Check sheet for the modelled part. Datum: model origin and axes. Units: mm. Coordinates: 2 decimals unless noted, no trailing zeros. Write each loop counter-clockwise with the first axis right and the second up, starting at its lowest first coordinate (ties: lowest second). Pieces come first, ordered by that corner, then holes. Notation, with made-up numbers: M -31,10.25 L 2,10.25 A22 ccw 2,49.25 Z; hole C 45,64 d10. An arc over 180 degrees is marked long. Answer as CSV lines item,"result". Start each with the question number.
Q1. Sectioned sample at C-C, the plane x = -4.75. Record the cut outline in (y, z).
Q2. Thickness scan on line 1 along Z through (x, y) = (-4, 3.5); line 2 along X through (y, z) = (0, -30.5) (3 decimals). Record the ranges inside material, lowest first. Write a range as from..to.
Q3. Sectioned sample at B-B, the plane z = -45. Record the cut outline in (x, y) (3 decimals).
Q4. Sectioned sample at A-A, the plane y = 0. Record the cut outline in (x, z) (1 decimal).
Q5. Depth check by flat-ended pin: pin 1 Ø1.8 at (y, z) = (0.5, -1.5) entering from -X; pin 2 Ø4 at (y, z) = (3.5, -17) entering from -X; pin 3 Ø1.1 at (y, z) = (-0.5, -1.5) entering from +X. Enter the tip coordinate at first touch or a pass-through.
from build123d import *

# Parameters (mm, degrees)
SKETCH1_W          = 47.625
SKETCH1_H          = 3.175
CHAMFER1_SIZE      = 0.9525
CUT_EXTRUDE2_DEPTH = 2.34696


with BuildPart() as part:
    # Sketch1 → Revolve1 (revolve)
    with BuildSketch(Plane(origin=(0, 0, 0), x_dir=(0, 0, -1), z_dir=(1, 0, 0))):
        with Locations((27.1653, 1.5875)):
            Rectangle(SKETCH1_W, SKETCH1_H)
    revolve(axis=Axis((0, 0, -50.9778), (0, 0, 1)))

    # Chamfer1
    chamfer1_edges = [part.edges().sort_by_distance(p)[0] for p in [
        (0, -3.175, -50.9778),
    ]]
    chamfer(chamfer1_edges, length=CHAMFER1_SIZE)

    # Sketch7 → Revolve2 (revolve)
    with BuildSketch(Plane(origin=(0, 0, 0), x_dir=(0, 0, -1), z_dir=(1, 0, 0)), mode=Mode.PRIVATE) as revolve2_sk:
        with BuildLine():
            Line((2.84988, 5.5499), (3.3528, 5.5499))
            Line((3.3528, 5.5499), (3.3528, 0))
            Line((3.3528, 0), (0, 0))
            Line((0, 0), (0, 3.175))
            ThreePointArc((0, 3.175), (1.235921075, 4.58927271), (2.84988, 5.5499))
        make_face()
    revolve(revolve2_sk.sketch.rotate(Axis((0, 0, 0), (0, 0, -1)), 180), axis=Axis((0, 0, 0), (0, 0, -1)))

    # Sketch5 → Cut-Extrude2 (cut)
    with BuildSketch(Plane.XY):
        Polygon((1.984375, -1.14567944), (1.984375, 1.14567944), (0, 2.291358881), (-1.984375, 1.14567944), (-1.984375, -1.14567944), (0, -2.291358881), align=None)
    extrude(amount=-CUT_EXTRUDE2_DEPTH, mode=Mode.SUBTRACT)

    # Cut-Extrude3 cone 1 section (on through the dimple's axis) → Cut-Extrude3 (revolve, cut)
    with BuildSketch(Plane(origin=(0, 0, 0), x_dir=(0, -1, 0), z_dir=(1, 0, 0))):
        Polygon((0, 0), (2.291358881, 0), (0, 2.291358881), align=None)
    revolve(axis=Axis((0, 0, 0), (0, 0, -1)), mode=Mode.SUBTRACT)


solid = part.part
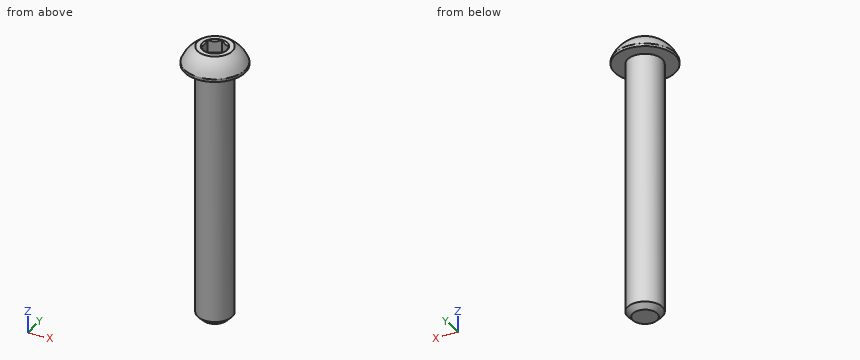
Output:
1,outline,"M -2.87,-3.35 L 2.87,-3.35 L 2.87,-2.85 A3.62 ccw -2.87,-2.85 Z"
2,line 1,"z = -3.35..-2.33"
2,line 2,"x = -3.175..3.175"
3,outline,"C 0,0 d6.35"
4,outline,"M -5.5,-3.4 L -3.2,-3.4 L -3.2,-50 L -2.2,-51 L 2.2,-51 L 3.2,-50 L 3.2,-3.4 L 5.5,-3.4 L 5.5,-2.8 A6 ccw 3.2,0 L 2.3,0 L 2,-0.3 L 2,-2.3 L -2,-2.3 L -2,-0.3 L -2.3,0 L -3.2,0 A6 ccw -5.5,-2.8 Z"
5,pin 1,"stops at x = -5.33"
5,pin 2,"stops at x = -2.8"
5,pin 3,"stops at x = 5.14"
